The listing builds one solid part. Answer for the finished solid, in the listing's coordinates (mm). A direction names the side the tool comes from. Coordinates: 2 decimals unless noted, no trailing zeros. Write each loop counter-clockwise with the first axis right and the second up, starting at its lowest first coordinate (ties: lowest second). Pieces come first, ordered by that corner, then holes. Notation, with made-up numbers: M -13.5,30.25 L 19.5,30.25 A16 cw 19.5,46.25 Z; hole C 68.25,10 d1. An arc over 180 degrees is marked long. Answer as CSV lines item,"result". Start each with the question number.
```python
from build123d import *

# Parameters (mm, degrees)
BOSS_EXTRUDE1_DEPTH = 5
SKETCH2_R           = 2.5
BOSS_EXTRUDE2_DEPTH = 7
SKETCH3_R           = 1
CUT_EXTRUDE1_DEPTH  = 5


with BuildPart() as part:
    # Sketch1 → Boss-Extrude1 (new body)
    with BuildSketch(Plane.XY):
        with BuildLine():
            Line((8.444274161, -42.5), (8.444274161, -23.602240521))
            Line((8.444274161, -23.602240521), (-13.047599403, -23.602240521))
            Line((-13.047599403, -23.602240521), (-21.798721118, -23.602240521))
            ThreePointArc((-21.798721118, -23.602240521), (-22.926788134, -22.508051578), (-24, -21.360009363))
            Line((-24, -21.360009363), (-39, -21.360009363))
            Line((-39, -21.360009363), (-39, -38.781438859))
            ThreePointArc((-39, -38.781438859), (55, 0), (-39, 38.781438859))
            Line((-39, 38.781438859), (-39, 21.360009363))
            Line((-39, 21.360009363), (-24, 21.360009363))
            ThreePointArc((-24, 21.360009363), (-22.926788134, 22.508051578), (-21.798721118, 23.602240521))
            Line((-21.798721118, 23.602240521), (8.444274161, 23.653441006))
            Line((8.444274161, 23.653441006), (8.444274161, 42.5))
            Line((8.444274161, 42.5), (24.94401824, 42.5))
            ThreePointArc((24.94401824, 42.5), (27.772445365, 41.328427125), (28.94401824, 38.5))
            Line((28.94401824, 38.5), (28.94401824, -38.5))
            ThreePointArc((28.94401824, -38.5), (27.772445365, -41.328427125), (24.94401824, -42.5))
            Line((24.94401824, -42.5), (8.444274161, -42.5))
        make_face()
    extrude(amount=BOSS_EXTRUDE1_DEPTH)

    # Sketch2 → Boss-Extrude2 (add)
    with BuildSketch(Plane(origin=(0, 0, 0), x_dir=(-1, 0, 0), z_dir=(0, 0, -1))):
        with Locations(Location((0, -33.5, 0), (0, 0, 180))):
            Circle(SKETCH2_R)
        with Locations(Location((0, 33.5, 0), (0, 0, 180))):
            Circle(SKETCH2_R)
    extrude(amount=BOSS_EXTRUDE2_DEPTH)

    # Sketch3 → Cut-Extrude1 (cut)
    with BuildSketch(Plane.XY.offset(5)):
        with Locations((-30.537878891, -34)):
            Circle(SKETCH3_R)
        with Locations((-30.537878891, 34)):
            Circle(SKETCH3_R)
        with Locations((47, 11)):
            Circle(SKETCH3_R)
        with Locations((47, -11)):
            Circle(SKETCH3_R)
    extrude(amount=-CUT_EXTRUDE1_DEPTH, mode=Mode.SUBTRACT)


solid = part.part
```
1) Each of these flat-tipped pins is pushed along its axis until it touches: P1, Ø1.5, axis at y = 8.5, z = 2.5, coming from the -X side; P2, Ø6, axis at y = -39.5, z = 1.5, coming from the -X side; P3, Ø5.5, axis at x = 0.5, z = 3.5, coming from the +Y side; P4, Ø3, axis at x = 47, y = 11, coming from the -Z side. Where does it stop, or does it pass through?
2) The part is cut by section C-C (y = 48). Determine the outline of the cut face in (x, z), then the cut area to 3 significant figures.
3) The part is cut by section B-B (x = -11). Determine the outline of the cut face in (y, z), then the cut area to 3 significant figures.
4) Find the intervals of material crossed by line 1 (Y direction, x = 47, z = 3.7); line 2 (Z direction, x = 11, y = -49); line 3 (Y direction, x = -7.5, z = 1.25), in increasing order. Write a range as from..to.
5) The part is cut by section D-D (x = 42). Determine the outline of the cut face in (y, z), then the cut area to 3 significant figures.
6) The part is cut by section A-A (x = 5). Determine the outline of the cut face in (y, z), then the cut area to 3 significant figures.
7) For a pull along X with two mould halves and no side action, classify faces 1 (the face through (28.944, 1, 2)), 2 (the face through (-22.911, -22.524, 2.465)), 3 (the face through (-39, 30, 2)), 4 (the face through (7, -24, 5)) as +X half, -X half, draft (parallel to the pull), parting line (faces both ways), or undercut.
8) Which of the six approach directions +Z, -Z, +X, -X, +Y, -Y give full straight-line access (tool end or side, diameter ignored) to faces 5 (the face through (-31, -21.36, 2)), 6 (the face through (1.34, -35.61, -3.45)), 7 (the face through (8.444, -33, 2))?
Completed:
1,P1,"x = 28.94"
1,P2,"x = -39"
1,P3,"y = 55"
1,P4,"z = 0"
2,outline,"M -26.85,0 L 26.85,0 L 26.85,5 L -26.85,5 Z"
2,area,"269 mm²"
3,outline,"M -53.89,0 L -23.6,0 L -23.6,5 L -53.89,5 Z; M 23.62,0 L 53.89,0 L 53.89,5 L 23.62,5 Z"
3,area,"303 mm²"
4,line 1,"-28.57..-12, -10..10, 12..28.57"
4,line 2,"0..5"
4,line 3,"-54.49..-23.6, 23.63..54.49"
5,outline,"M -35.51,0 L 35.51,0 L 35.51,5 L -35.51,5 Z"
5,area,"355 mm²"
6,outline,"M -54.77,0 L -23.6,0 L -23.6,5 L -54.77,5 Z; M 23.65,0 L 54.77,0 L 54.77,5 L 23.65,5 Z"
6,area,"311 mm²"
7,face 1,"undercut"
7,face 2,"undercut"
7,face 3,"-X half"
7,face 4,"draft"
8,face 5,"+Z, -Z, -X"
8,face 6,"-Z"
8,face 7,"+Z, -Z"
